from build123d import *

# Parameters (mm, degrees)
F0_R     = 5
F1_DEPTH = 18
F4_D     = 7
F4_DEPTH = 35
F4_TIP   = 2.1030121666
F5_D     = 7
F5_DEPTH = 35
F5_TIP   = 2.1030121666
F6_R     = 15
F6_R_2   = 2.5
F7_DEPTH = 1


with BuildPart() as f1:
    # F0 (on Front) → F1 (new body)
    with BuildSketch(Plane.XZ):
        with BuildLine():
            Line((0, 70), (0, 0))
            Line((0, 0), (491, 0))
            Line((491, 0), (491, 70))
            Line((491, 70), (475.1421356237, 70))
            ThreePointArc((475.1421356237, 70), (471.3153013001, 69.2387953251), (468.0710678119, 67.0710678119))
            Line((468.0710678119, 67.0710678119), (446.8578643763, 45.8578643763))
            ThreePointArc((446.8578643763, 45.8578643763), (440.3693973998, 41.5224093498), (432.7157287525, 40))
            Line((432.7157287525, 40), (58.2842712475, 40))
            ThreePointArc((58.2842712475, 40), (50.6306026002, 41.5224093498), (44.1421356237, 45.8578643763))
            Line((44.1421356237, 45.8578643763), (22.9289321881, 67.0710678119))
            ThreePointArc((22.9289321881, 67.0710678119), (19.6846986999, 69.2387953251), (15.8578643763, 70))
            Line((15.8578643763, 70), (0, 70))
        make_face()
        with Locations((25, 19)):
            Circle(F0_R, mode=Mode.SUBTRACT)
        with Locations((466, 19)):
            Circle(F0_R, mode=Mode.SUBTRACT)
    extrude(amount=F1_DEPTH)

    # F4
    with Locations(Plane(origin=(0, 0, 0), x_dir=(0, -1, 0), z_dir=(-1, 0, 0))):
        with Locations((9, 19)):
            Hole(F4_D / 2, depth=F4_DEPTH)
            with Locations((0, 0, -(F4_DEPTH + F4_TIP / 2))):  # 118° drill point
                Cone(0, F4_D / 2, F4_TIP, mode=Mode.SUBTRACT)

    # F5
    with Locations(Plane.YZ.offset(491)):
        with Locations((-9, 19)):
            Hole(F5_D / 2, depth=F5_DEPTH)
            with Locations((0, 0, -(F5_DEPTH + F5_TIP / 2))):  # 118° drill point
                Cone(0, F5_D / 2, F5_TIP, mode=Mode.SUBTRACT)

    # F6 (on face) → F7 (cut)
    with BuildSketch(Plane.XZ.offset(18)):
        with Locations((245.5, 20.5260608345)):
            Circle(F6_R)
        with Locations((244.5451939106, 12.0426760986)):
            Circle(F6_R_2, mode=Mode.SUBTRACT)
        Polygon((242.0451939106, 16.5260608345), (242.0451939106, 28.5260608345), (246.0451939106, 28.5260608345), (246.0451939106, 20.5260608345), (252.542167902, 20.5260608345), (252.542167902, 16.5260608345), align=None, mode=Mode.SUBTRACT)
    extrude(amount=-F7_DEPTH, mode=Mode.SUBTRACT)


solid = f1.part
Can you work these out from the model? Positions are in its coordinate system, mm. A direction names the side the tool comes from. Round coordinates to 2 decimals unless told otherwise and drop trailing zeros. Order: outer loops, then holes, each group sorted by start corner. A loop starts at its lowest first (then second) coordinate and runs counter-clockwise, first axis right, second up. Notation, with made-up numbers: (85, -10.5) - (101, -10.5) arc R10 cw to (101, -4.5) - close; hole circle Ø10 at (20, 57.25). An arc over 180 degrees is marked (long way). Answer in a Markdown table with one row per item.
(1) Which directions (+Z, -Z, +X, -X, +Y, -Y) give clear straight access to the entire face, cutting with the end or side of a thin tool? Please do faces 1 (the face through (259.356, -17.507, 14.781)), 2 (the face through (248, -9, 40)), 3 (the face through (464.92, -8.87, 14.12)).
From the geometry:
| item | result |
|---|---|
| face 1 | -Y |
| face 2 | +Z, +Y, -Y |
| face 3 | +Y, -Y |
(2) Please list where these lines run through material, in increasing order: L1, parallel to X at y = -15.25, z = 19; L2, parallel to Y at x = 5, z = 19; L3, parallel to X at y = -8, z = 61.5. Write a range as from..to.
From the geometry:
| item | result |
|---|---|
| L1 | x = 0..20, 30..461, 471..491 |
| L2 | y = -18..-12.5, -5.5..0 |
| L3 | x = 0..28.5, 462.5..491 |
(3) If we mould it in two halves opening along X, with no side actions, what happens to faces 4 (the face through (245, -18, 21)), 5 (the face through (34, -9, 56)), 6 (the face through (0, -9, 35))? For each: released by +X, released by -X, zero draft, split by the parting line, or undercut.
From the geometry:
| item | result |
|---|---|
| face 4 | zero draft |
| face 5 | undercut |
| face 6 | released by -X |
(4) For P1, Ø5, axis at x = 245.5, y = -7, coming from the +Z side; P2, Ø6, axis at x = 25, z = 19, coming from the -Y side; P3, Ø5.5, axis at y = -9, z = 19, coming from the -X side; P4, Ø5.5, axis at y = -9, z = 19, coming from the +X side, each with a flat end and sliding along its axis, tell me the tip position at first contact or that it passes through.
From the geometry:
| item | result |
|---|---|
| P1 | stops at z = 40 |
| P2 | passes through |
| P3 | stops at x = 35.45 |
| P4 | stops at x = 455.55 |
(5) Suppose I cut it at A-A, the plane x = 334.5. Please give me the cut outline in (y, z).
From the geometry:
| item | result |
|---|---|
| outline | (-18, 0) - (0, 0) - (0, 40) - (-18, 40) - close |
